```python
from build123d import *

# Parameters (mm, degrees)
SKETCH1_W           = 26.999950409
SKETCH1_H           = 3
BOSS_EXTRUDE1_DEPTH = 12
CUT_EXTRUDE1_DEPTH  = 11.5
BOSS_EXTRUDE2_DEPTH = 1
SKETCH7_R           = 0.7
CUT_EXTRUDE2_DEPTH  = 6
SKETCH8_R           = 1.549809906
BOSS_EXTRUDE3_DEPTH = 2
SKETCH11_W          = 30.763753833
SKETCH11_H          = 8
CUT_EXTRUDE3_DEPTH  = 1.2
FILLET1_R           = 1
SKETCH12_R          = 3.153602023
CUT_EXTRUDE4_DEPTH  = 10
CUT_EXTRUDE5_DEPTH  = 2
SKETCH14_R          = 0.7
BOSS_EXTRUDE4_DEPTH = 1


with BuildPart() as part:
    # Sketch1 → Boss-Extrude1 (new body)
    with BuildSketch(Plane(origin=(0, 0, 0), x_dir=(1, 0, 0), z_dir=(0, 1, 0))):
        with Locations((-4.128207024, 7.928244269)):
            Rectangle(SKETCH1_W, SKETCH1_H)
        Polygon((7.371810524, -11.571754957), (7.371810524, 4.428244174), (-15.628224572, 4.428244174), (-15.628224572, -11.571754957), (-15.728224572, -11.571754957), (-20.628203209, -11.571754957), (-20.628203209, -9.571756491), (-17.628182229, -7.119161332), (-17.628182229, 6.428244269), (9.37176818, 6.428244269), (9.37176818, -2.571755344), (12.371848766, -9.571756491), (12.371848766, -11.571754957), (7.471810524, -11.571754957), align=None)
    extrude(amount=BOSS_EXTRUDE1_DEPTH)

    # Sketch4 → Cut-Extrude1 (cut)
    with BuildSketch(Plane(origin=(12.371848766, 0, 0), x_dir=(0, 0, -1), z_dir=(1, 0, 0))):
        Polygon((4.428244174, 0), (4.428244174, 8.000016212), (-1.618738598, 8.000016212), (-9.571756491, 0), (-11.571754957, 0), align=None)
    extrude(amount=-CUT_EXTRUDE1_DEPTH, mode=Mode.SUBTRACT)

    # Sketch5 → Boss-Extrude2 (add)
    with BuildSketch(Plane(origin=(0, 12, 0), x_dir=(1, 0, 0), z_dir=(0, 1, 0))):
        Polygon((-20.628203209, -9.571756491), (-20.628203209, -11.571754957), (12.371848766, -11.571754957), (12.371848766, -9.571756491), (9.37176818, -2.571755344), (9.37176818, 9.428244269), (-17.628182229, 9.428244269), (-17.628182229, -7.119161332), align=None)
    extrude(amount=BOSS_EXTRUDE2_DEPTH)

    # Sketch7 → Cut-Extrude2 (cut)
    with BuildSketch(Plane.XY.offset(11.571754957)):
        with Locations((-18.144630941, 5.602586011)):
            Circle(SKETCH7_R)
        with Locations((10.055363141, 5.602566371)):
            Circle(SKETCH7_R)
    extrude(amount=-CUT_EXTRUDE2_DEPTH, mode=Mode.SUBTRACT)

    # Sketch8 → Boss-Extrude3 (add)
    with BuildSketch(Plane(origin=(0, 0, -9.428244269), x_dir=(-1, 0, 0), z_dir=(0, 0, -1))):
        with BuildLine():
            ThreePointArc((7.167350646, 16.881210895), (4.06111535, 20.071343328), (0.789350976, 17.051210792))
            Line((0.789350976, 17.051210792), (0.801312783, 15.286719843))
            ThreePointArc((0.801312783, 15.286719843), (0.398304036, 13.90328737), (-0.724359486, 13))
            Line((-0.724359486, 13), (8.821641956, 13))
            ThreePointArc((8.821641956, 13), (7.624453215, 13.872256527), (7.167350646, 15.281209887))
            Line((7.167350646, 15.281209887), (7.167350646, 16.881210895))
        make_face()
        with Locations((4.030375515, 16.793532247)):
            Circle(SKETCH8_R, mode=Mode.SUBTRACT)
        with BuildLine():
            Line((8.821641956, 0), (-0.724359486, 0))
            ThreePointArc((-0.724359486, 0), (0.554106373, -1.994843204), (0.893224509, -4.339810848))
            Line((0.893224509, -4.339810848), (0.881225349, -6.109811753))
            ThreePointArc((0.881225349, -6.109811753), (4.004145214, -8.784221579), (7.170605746, -6.16150846))
            Line((7.170605746, -6.16150846), (7.170605746, -4.561507453))
            ThreePointArc((7.170605746, -4.561507453), (7.476553675, -2.092695462), (8.821641956, 0))
        make_face()
        with Locations((4.030375515, -5.593063946)):
            Circle(SKETCH8_R, mode=Mode.SUBTRACT)
    extrude(amount=-BOSS_EXTRUDE3_DEPTH)

    # Sketch11 → Cut-Extrude3 (cut)
    with BuildSketch(Plane(origin=(0, 0, -9.428244269), x_dir=(-1, 0, 0), z_dir=(0, 0, -1))):
        with Locations((4.128177222, 6.5)):
            Rectangle(SKETCH11_W, SKETCH11_H)
    extrude(amount=-CUT_EXTRUDE3_DEPTH, mode=Mode.SUBTRACT)

    # Fillet1
    fillet1_edges = [part.edges().sort_by_distance(p)[0] for p in [
        (-4.048641235, 13, -7.428244269),
        (-4.048641235, 0, -7.428244269),
    ]]
    fillet(fillet1_edges, radius=FILLET1_R)

    # Sketch12 → Cut-Extrude4 (cut)
    with BuildSketch(Plane.XY.offset(-7.428244269)):
        with Locations((-4.030375515, 16.793532247)):
            Circle(SKETCH12_R)
    extrude(amount=CUT_EXTRUDE4_DEPTH, mode=Mode.SUBTRACT)

    # Sketch13 → Cut-Extrude5 (cut)
    with BuildSketch(Plane.XY.offset(-4.428244174)):
        Polygon((-15.628224572, 0), (-15.628224572, 12), (7.371810524, 12), (7.371810524, 8.000016212), (9.37176818, 8.000016212), (9.37176818, 0), (7.371810524, 0), align=None)
    extrude(amount=-CUT_EXTRUDE5_DEPTH, mode=Mode.SUBTRACT)

    # Sketch14 → Boss-Extrude4 (add)
    with BuildSketch(Plane.XY.offset(11.571754957)):
        Polygon((-20.628203209, 0), (-20.628203209, 13), (12.371848766, 13), (12.371848766, 0), (7.371810524, 0), (7.371810524, 12), (-15.628224572, 12), (-15.628224572, 0), align=None)
        with Locations((-18.144630941, 5.602586011)):
            Circle(SKETCH14_R, mode=Mode.SUBTRACT)
        with Locations((10.055363141, 5.602566371)):
            Circle(SKETCH14_R, mode=Mode.SUBTRACT)
    extrude(amount=BOSS_EXTRUDE4_DEPTH)


solid = part.part
```
For this review, take the finished solid that the model builds, in its own axes (mm). A direction names the side the tool comes from. Give positions to 0.01 mm unless a question says otherwise; leave off trailing zeros. Write each loop counter-clockwise with the first axis right and the second up, starting at its lowest first coordinate (ties: lowest second). Pieces come first, ordered by that corner, then holes. Notation, with made-up numbers: M -38.75,62 L 3.25,62 A8 cw 3.25,72 Z; hole C 32,-8 d10. An arc over 180 degrees is marked long. Answer as a JSON object with one key per item and string values. Group by question number.
Item 1: For probe 1 along Z at (x, y) = (-10, 6.5); probe 2 along Y at (x, z) = (-10, 0); probe 3 along X at (y, z) = (4, 11), list the stretches that pass through material, from the lowest coordinate up. Write a range as [from, to].
Item 2: Consider section B-B on z = 10.5. Write out the cut boundary in (x, y).
Item 3: Consider section A-A on x = 6. Write out the cut boundary in (y, z), plus the area to 3 significant figures.
Item 4: Tool access review of faces 4 (the flat face through (8, 8, -2)), 5 (the flat face through (-7.167, 16, -8)), 6 (the flat face through (-4, 2.5, -9)), 7 (the flat face through (-5, -4, -7.428)), 8 (the flat face through (9.372, 9, -5)): name each direction out of +Z, -Z, +X, -X, +Y, -Y from which nothing blocks a thin tool from reaching the whole face with its end or side.
Item 5: Consider section D-D on y = 1.5. Write out the cut boundary in (x, z).
Item 6: Consider section C-C on z = -1. Write out the cut boundary in (x, y), plus the area to 3 significant figures.
Item 7: Draft analysis for pull direction Z (two halves, no side actions). For faces 1 (the flat face through (-4.1, 12.8, 12.572)), 2 (the flat face through (-16, 0, 0)), 3 (the flat face through (9.35, 3.17, 6.42)), state which applies: +Z half, -Z half, draft (parallel to the pull), parting line (faces both ways), or undercut.
Item 8: For pin 1 Ø3.5 at (x, z) = (10, 10.5) entering from -Y; pin 2 Ø8 at (x, y) = (-11, -2.5) entering from -Z; pin 3 Ø0.8 at (y, z) = (15.5, -8.5) entering from -X; pin 4 Ø5 at (x, z) = (-4.5, 1) entering from -Y, all flat-tipped, find the tip position at first contact; note any pin that passes through.
Check result:
{
 "1": {"probe 1": "z = [-8.23, -6.43]", "probe 2": "y = [12, 13]", "probe 3": "x = [-20.63, -15.63], [7.37, 12.37]"},
 "2": {"outline": "M -20.63,0 L -15.63,0 L -15.63,12 L 7.37,12 L 7.37,0 L 12.37,0 L 12.37,13 L -20.63,13 Z; hole C -18.14,5.6 d1.4; hole C 10.06,5.6 d1.4"},
 "3": {"outline": "M 0,-9.43 L 2.5,-9.43 L 2.5,-8.23 L 10.5,-8.23 L 10.5,-9.43 L 13,-9.43 L 13,12.57 L 12,12.57 L 12,-6.43 L 0,-6.43 Z", "area": "48.4 mm^2"},
 "4": {"face 4": "+X, -Y", "face 5": "+Z, -Z, -X, +Y", "face 6": "-Z, +X, -X", "face 7": "+Z, +X, -X, -Y", "face 8": "-Z, +X, +Y, -Y"},
 "5": {"outline": "M -20.63,9.57 L -17.63,7.12 L -17.63,-9.43 L 9.37,-9.43 L 9.37,-6.43 L -15.63,-6.43 L -15.63,12.57 L -20.63,12.57 Z; M 7.37,8.08 L 11.73,8.08 L 12.37,9.57 L 12.37,12.57 L 7.37,12.57 Z"},
 "6": {"outline": "M -17.63,0 L -15.63,0 L -15.63,12 L 7.37,12 L 7.37,8 L 9.37,8 L 9.37,13 L -17.63,13 Z", "area": "59.0 mm^2"},
 "7": {"face 1": "+Z half", "face 2": "draft", "face 3": "undercut"},
 "8": {"pin 1": "stops at y = 0", "pin 2": "stops at z = -9.43", "pin 3": "stops at x = -7.17", "pin 4": "stops at y = 12"}
}
